Build history of the part. All positions in model axes, mm. A direction names the side the tool comes from. Round coordinates to 2 decimals unless told otherwise and drop trailing zeros. Write each loop counter-clockwise with the first axis right and the second up, starting at its lowest first coordinate (ties: lowest second). Pieces come first, ordered by that corner, then holes. Notation, with made-up numbers: M -19,-13 L 19,-13 A18 ccw 19,-1 Z; hole C 65,10 d9. An arc over 180 degrees is marked long. Write item = value, one per line.
from build123d import *

# Parameters (mm, degrees)
F0_R      = 14.9225
F1_DEPTH  = 7.62
F2_R      = 11.0236
F3_DEPTH  = 25.4
F5_DEPTH  = 6.35
F6_R      = 14.9225
F7_DEPTH  = 6.35
F8_R      = 11.0236
F9_DEPTH  = 25.4
F10_R     = 11.0236
F11_DEPTH = 25.4
F12_R     = 11.0236
F13_DEPTH = 25.4
F14_R     = 11.0236
F15_DEPTH = 25.4


with BuildPart() as f1:
    # F0 (on Top) → F1 (new body)
    with BuildSketch(Plane.XY):
        Circle(F0_R)
    extrude(amount=F1_DEPTH)

    # F2 (on face) → F3 (cut)
    with BuildSketch(Plane.XY.offset(7.62)):
        Circle(F2_R)
    extrude(amount=-F3_DEPTH, mode=Mode.SUBTRACT)

    # F4 (on Top) → F5 (join)
    with BuildSketch(Plane.XY):
        Polygon((23.40718, 3.830266), (14.89548, 3.830266), (14.611755, -2.979096), (23.40718, -2.979096), align=None)
        Polygon((-3.275654, 23.123458), (-3.275654, 14.611758), (3.533708, 14.328033), (3.533708, 23.123458), align=None)
        Polygon((-14.23008, 3.830266), (-22.74178, 3.830266), (-23.025505, -2.979096), (-14.23008, -2.979096), align=None)
        Polygon((4.597669, -23.888158), (4.597669, -15.057278), (-3.062862, -14.773545), (-3.062862, -23.888158), align=None)
    extrude(amount=F5_DEPTH)

    # F6 (on Top) → F7 (join)
    with BuildSketch(Plane.XY):
        with Locations((37.025906, 0)):
            Circle(F6_R)
        with Locations((0, 37.025906)):
            Circle(F6_R)
        with Locations((-36.742181, 0)):
            Circle(F6_R)
        with Locations((0, -37.877075)):
            Circle(F6_R)
    extrude(amount=F7_DEPTH)

    # F8 (on face) → F9 (cut)
    with BuildSketch(Plane.XY.offset(6.35)):
        with Locations((-36.742181, 0)):
            Circle(F8_R)
    extrude(amount=-F9_DEPTH, mode=Mode.SUBTRACT)

    # F10 (on face) → F11 (cut)
    with BuildSketch(Plane.XY.offset(6.35)):
        with Locations((0, 37.025906)):
            Circle(F10_R)
    extrude(amount=-F11_DEPTH, mode=Mode.SUBTRACT)

    # F12 (on face) → F13 (cut)
    with BuildSketch(Plane.XY.offset(6.35)):
        with Locations((37.025906, 0)):
            Circle(F12_R)
    extrude(amount=-F13_DEPTH, mode=Mode.SUBTRACT)

    # F14 (on face) → F15 (cut)
    with BuildSketch(Plane.XY.offset(6.35)):
        with Locations((0, -37.877075)):
            Circle(F14_R)
    extrude(amount=-F15_DEPTH, mode=Mode.SUBTRACT)


solid = f1.part
1. Band-saw the part on A-A (y = 0). List the corners of the cut face in (x, z), plus the area to 3 significant figures.
Responses:
outline = M -51.66,0 L -47.77,0 L -47.77,6.35 L -51.66,6.35 Z; M -25.72,0 L -11.02,0 L -11.02,7.62 L -14.92,7.62 L -14.92,6.35 L -25.72,6.35 Z; M 11.02,0 L 26,0 L 26,6.35 L 14.92,6.35 L 14.92,7.62 L 11.02,7.62 Z; M 48.05,0 L 51.95,0 L 51.95,6.35 L 48.05,6.35 Z
area = 248 mm²
2. Flat gauge pins, fed straight in: pin 1 (4 mm diameter, centred on y = 18, z = 2.5, fed in from -X); pin 2 (1.9 mm diameter, centred on x = 20, z = 2, fed in from +Y); pin 3 (17.5 mm diameter, centred on x = 0, y = -37.88, fed in from -Z); pin 4 (9 mm diameter, centred on x = 5, y = 25.5, fed in from +Z). Where does each tip first touch, or does it go through?
Responses:
pin_1 = -3.28
pin_2 = 3.83
pin_3 = through
pin_4 = 6.35
3. Tool access for faces 1 (the face through (19, 3.83, 3)), 2 (the face through (-7, -9, 7.62)): list every direction of +Z, -Z, +X, -X, +Y, -Y with a clear straight run to the whole face (end or side of a thin tool).
Responses:
face_1 = +Z, -Z, +Y
face_2 = +Z, +X, -X, +Y, -Y
4. Band-saw the part on B-B (y = 27.5). List the corners of the cut face in (x, z).
Responses:
outline = M -11.49,0 L -5.55,0 L -5.55,6.35 L -11.49,6.35 Z; M 5.55,0 L 11.49,0 L 11.49,6.35 L 5.55,6.35 Z
5. Band-saw the part on C-C (x = -33.5). List the corners of the cut face in (y, z), plus the area to 3 significant figures.
Responses:
outline = M -14.57,0 L -10.54,0 L -10.54,6.35 L -14.57,6.35 Z; M 10.54,0 L 14.57,0 L 14.57,6.35 L 10.54,6.35 Z
area = 51.2 mm²
6. Band-saw the part on D-D (z = 2.75). Count the separate pieces of the cut face and the enclosed holes in it, plus the area to 3 significant figures.
Responses:
separate_pieces = 1
enclosed_holes = 5
area = 1,800 mm²
7. Probe probe 1 along Y at (x, z) = (0, 2.5); probe 2 along Y at (x, z) = (5, 2.25); probe 3 along X at (y, z) = (-38.5, 5.75). List the from-to ranges inside material, lowest first.
Responses:
probe_1 = -52.8 to -48.9, -26.85 to -11.02, 11.02 to 26, 48.05 to 51.95
probe_2 = -51.94 to -47.7, -28.05 to -23.82, -14.06 to -9.82, 9.82 to 14.06, 22.97 to 27.2, 46.85 to 51.09
probe_3 = -14.91 to -11.01, 11.01 to 14.91
8. Mould opens along Y. For faces 3 (the face through (-3, 26, 6.35)), 4 (the face through (3.534, 18, 3)), 5 (the face through (-51.664, 0.171, 3.131)) say: pulls with the +Y half, pulls with the -Y half, needs draft (parallel to the pull), parting line crosses it, or undercut.
Responses:
face_3 = needs draft
face_4 = undercut
face_5 = parting line crosses it
